```python
from build123d import *

# Parameters (mm, degrees)
F0_W     = 71.80331
F0_H     = 62.466614
F1_DEPTH = 7.62
F0_W_2   = 86.302102
F0_H_2   = 76.759144
F2_DEPTH = 76.2


with BuildPart() as f1:
    # F0 (on Front) → F1 (new body)
    with BuildSketch(Plane.XZ):
        Rectangle(F0_W, F0_H)
    extrude(amount=F1_DEPTH)

    # F0 (on Front) → F2 (join)
    with BuildSketch(Plane.XZ):
        Rectangle(F0_W_2, F0_H_2)
        Rectangle(F0_W, F0_H, mode=Mode.SUBTRACT)
    extrude(amount=F2_DEPTH)


solid = f1.part
```
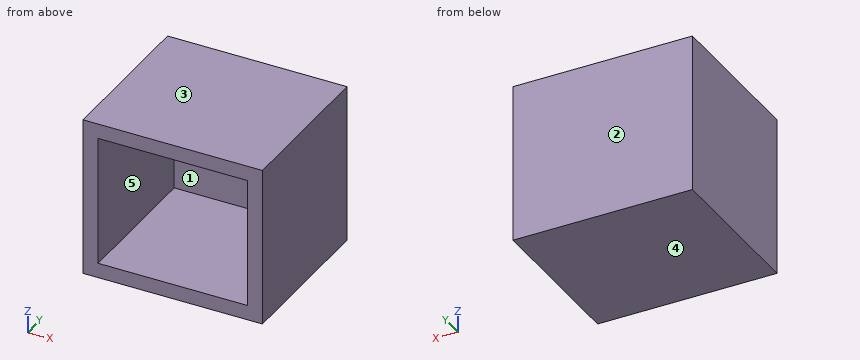
Geometry: final body of the model. Coordinates: model frame, mm. Face numbers are marked on the shaded views. A direction names the side the tool comes from. Round coordinates to 2 decimals unless told otherwise and drop trailing zeros. Order: outer loops, then holes, each group sorted by start corner. A loop starts at its lowest first (then second) coordinate and runs counter-clockwise, first axis right, second up. Notation, with made-up numbers: (74.5, -1) - (98.5, -1) arc R14 cw to (98.5, 25) - close; hole circle Ø5 at (77, -30). An arc over 180 degrees is marked (long way). Use CSV: the item, a comma, the result in double quotes. Start each with the question number.
Q1. Material intervals for line 1 along Z through (x, y) = (-26, -8); line 2 along X through (y, z) = (-58, -7.5); line 3 along Y through (x, z) = (-0.5, -17.5), sorted ascending. Write a range as from..to.
Q2. Access query for the marked faces 1 and 2. Directions: +Z, -Z, +X, -X, +Y, -Y. A direction counts if a zero-diameter tool reaches every point of the face in a straight line with its end or side. Return the directions, or none.
Q3. Mould query, pull axis Z, two halves, no side actions, for the marked faces 3, 4 and 5. Classes: +Z half, -Z half, draft (parallel to the pull), parting line (faces both ways), or undercut.
Q4. Section query C-C (x = 21). Return loops of the section in (y, z).
Q5. First-contact query: pin 1 (18.5 mm diameter, centred on x = 5, z = -0.5, fed in from -Y); pin 2 (8 mm diameter, centred on x = 18, z = -6, fed in from +Y). Flat tips, straight axial feed; report the tip coordinate or a pass-through.
Q6. Section query A-A (y = -12). Return loops of the section in (x, z), and give its area (3 significant figures).
Q7. Section query B-B (z = 5). Return loops of the section in (x, y).
Result set:
1,line 1,"z = -38.38..-31.23, 31.23..38.38"
1,line 2,"x = -43.15..-35.9, 35.9..43.15"
1,line 3,"y = -7.62..0"
2,face 1,"-Y"
2,face 2,"+Z, -Z, +X, -X, +Y"
3,face 3,"+Z half"
3,face 4,"-Z half"
3,face 5,"undercut"
4,outline,"(-76.2, -38.38) - (0, -38.38) - (0, 38.38) - (-76.2, 38.38) - (-76.2, 31.23) - (-7.62, 31.23) - (-7.62, -31.23) - (-76.2, -31.23) - close"
5,pin 1,"stops at y = -7.62"
5,pin 2,"stops at y = 0"
6,outline,"(-43.15, -38.38) - (43.15, -38.38) - (43.15, 38.38) - (-43.15, 38.38) - close; hole (-35.9, -31.23) - (35.9, -31.23) - (35.9, 31.23) - (-35.9, 31.23) - close"
6,area,"2,140 mm2"
7,outline,"(-43.15, -76.2) - (-35.9, -76.2) - (-35.9, -7.62) - (35.9, -7.62) - (35.9, -76.2) - (43.15, -76.2) - (43.15, 0) - (-43.15, 0) - close"
